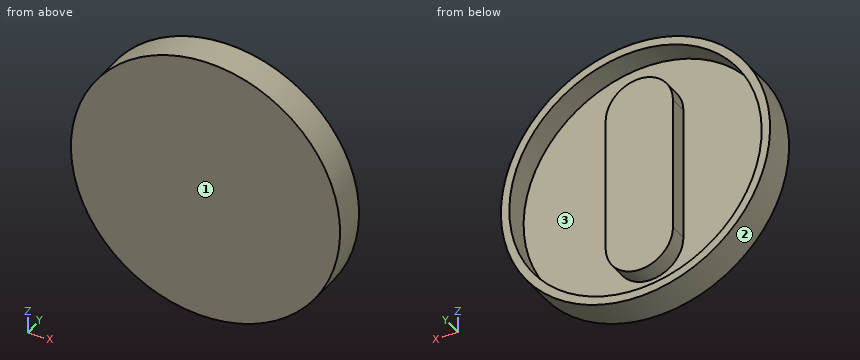
from build123d import *

# Parameters (mm, degrees)
SKETCH1_R           = 101.6
BOSS_EXTRUDE1_DEPTH = 25.4
SKETCH3_R           = 95.25
CUT_EXTRUDE1_DEPTH  = 19.05
BOSS_EXTRUDE2_DEPTH = 13.97


with BuildPart() as part:
    # Sketch1 → Boss-Extrude1 (new body)
    with BuildSketch(Plane(origin=(0, 0, 0), x_dir=(1, 0, 0), z_dir=(0, 1, 0))):
        with Locations(Location((0, 0, 0), (0, 0, 270))):
            Circle(SKETCH1_R)
    extrude(amount=BOSS_EXTRUDE1_DEPTH)

    # Sketch3 → Cut-Extrude1 (cut)
    with BuildSketch(Plane(origin=(0, 25.4, 0), x_dir=(1, 0, 0), z_dir=(0, 1, 0))):
        with Locations(Location((0, 0, 0), (0, 0, 270))):
            Circle(SKETCH3_R)
    extrude(amount=-CUT_EXTRUDE1_DEPTH, mode=Mode.SUBTRACT)

    # Sketch5 → Boss-Extrude2 (add)
    with BuildSketch(Plane(origin=(0, 6.35, 0), x_dir=(1, 0, 0), z_dir=(0, 1, 0))):
        with BuildLine():
            Line((-25.4, -50.707939874), (-25.4, 50.707939874))
            ThreePointArc((-25.4, 50.707939874), (0, 76.107939874), (25.4, 50.707939874))
            Line((25.4, 50.707939874), (25.4, -50.707939874))
            ThreePointArc((25.4, -50.707939874), (0, -76.107939874), (-25.4, -50.707939874))
        make_face()
    extrude(amount=BOSS_EXTRUDE2_DEPTH)


solid = part.part
Read the model definition and answer for the solid it produces. Units are mm, in the model's axes. Face numbers are marked on the shaded views. Give positions to 0.01 mm unless a question says otherwise; leave off trailing zeros. Write each loop counter-clockwise with the first axis right and the second up, starting at its lowest first coordinate (ties: lowest second). Pieces come first, ordered by that corner, then holes. Notation, with made-up numbers: (-29.75, 51) -> (21.25, 51) arc R5 ccw to (21.25, 60) -> close; hole circle Ø10 at (-40, 1.5). An arc over 180 degrees is marked (long way). Answer as a JSON object with one key per item and string values. Group by question number.
1) Consider L1, parallel to X at y = 10.5, z = 0; L2, parallel to X at y = 21, z = 0; L3, parallel to X at y = 7, z = 27. Determine where each line is inside the solid, lowest interval first. Write a range as from..to.
2) Find section B-B (z = 0). Write down the section's boundary in (x, y), and give its area (3 significant figures).
3) Find section A-A (y = 13). Write down the section's boundary in (x, z).
4) Find section D-D (x = -31.5). Write down the section's boundary in (y, z).
5) Find section C-C (x = 0). Write down the section's boundary in (y, z), and give its area (3 significant figures).
6) The mould has two halves that part along Z. Classify the marked faces 1, 2 and 3: +Z half, -Z half, draft (parallel to the pull), parting line (faces both ways), or undercut.
7) Each of these flat-tipped pins is pushed along its axis until it touches: P1, Ø4, axis at y = 10, z = 8, coming from the -X side; P2, Ø4, axis at x = -63.5, y = 6, coming from the -Z side; P3, Ø5, axis at x = -53, y = 21.5, coming from the +Z side. Where does it stop, or does it pass through?
Values follow:
{
 "1": {"L1": "x = -101.6..-95.25, -25.4..25.4, 95.25..101.6", "L2": "x = -101.6..-95.25, 95.25..101.6", "L3": "x = -97.95..-91.34, -25.4..25.4, 91.34..97.95"},
 "2": {"outline": "(-101.6, 0) -> (101.6, 0) -> (101.6, 25.4) -> (95.25, 25.4) -> (95.25, 6.35) -> (25.4, 6.35) -> (25.4, 20.32) -> (-25.4, 20.32) -> (-25.4, 6.35) -> (-95.25, 6.35) -> (-95.25, 25.4) -> (-101.6, 25.4) -> close", "area": "2,240 mm2"},
 "3": {"outline": "circle Ø203.2 at (0, 0); (-25.4, -50.71) arc R25.4 ccw to (25.4, -50.71) -> (25.4, 50.71) arc R25.4 ccw to (-25.4, 50.71) -> close; hole circle Ø190.5 at (0, 0)"},
 "4": {"outline": "(0, -96.59) -> (25.4, -96.59) -> (25.4, -89.89) -> (6.35, -89.89) -> (6.35, 89.89) -> (25.4, 89.89) -> (25.4, 96.59) -> (0, 96.59) -> close"},
 "5": {"outline": "(0, -101.6) -> (25.4, -101.6) -> (25.4, -95.25) -> (6.35, -95.25) -> (6.35, -76.11) -> (20.32, -76.11) -> (20.32, 76.11) -> (6.35, 76.11) -> (6.35, 95.25) -> (25.4, 95.25) -> (25.4, 101.6) -> (0, 101.6) -> close", "area": "3,660 mm2"},
 "6": {"face 1": "draft", "face 2": "parting line", "face 3": "undercut"},
 "7": {"P1": "stops at x = -101.42", "P2": "stops at z = -80.87", "P3": "stops at z = 88.16"}
}
